Design review of the part built by this model. Coordinates are the model's own, in mm. Face numbers are marked on the shaded views. Round coordinates to 2 decimals unless told otherwise and drop trailing zeros. Loops run counter-clockwise (first coordinate to the right, second up) from the corner with the lowest first, then second, coordinate; pieces in that order, holes last. Notation, with made-up numbers: (-32, 4.25) -> (-20, 4.25) arc R13 cw to (-20, 9.25) -> close; hole circle Ø3 at (46, 52). An arc over 180 degrees is marked (long way). Write each question's results on one line, items separated by ' | '. Start each with the question number.
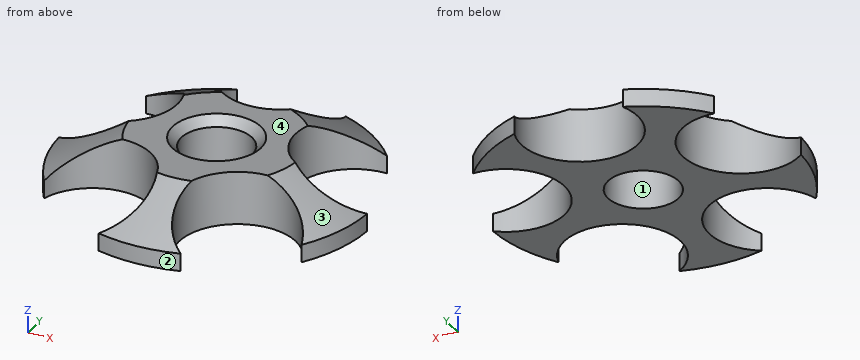
from build123d import *

# Parameters (mm, degrees)
F0_R     = 2
F1_DEPTH = 3
F2_SIZE2 = 2
F2_SIZE  = 4
F3_SIZE  = 0.5


with BuildPart() as f1:
    # F0 (on Top) → F1 (new body)
    with BuildSketch(Plane.XY):
        with BuildLine():
            ThreePointArc((-6.8389636709, 5.4581201808), (-3.5189091103, 1.1433628792), (-8.7410403812, -0.3958699968))
            ThreePointArc((-8.7410403812, -0.3958699968), (-8.3217445176, -2.7038987008), (-7.3043367629, -4.8175890707))
            ThreePointArc((-7.3043367629, -4.8175890707), (-2.1748054335, -2.9933628792), (-2.3246352862, -8.4355539703))
            ThreePointArc((-2.3246352862, -8.4355539703), (0, -8.75), (2.3246352862, -8.4355539703))
            ThreePointArc((2.3246352862, -8.4355539703), (2.1748054335, -2.9933628792), (7.3043367629, -4.8175890707))
            ThreePointArc((7.3043367629, -4.8175890707), (8.3217445176, -2.7038987008), (8.7410403812, -0.3958699968))
            ThreePointArc((8.7410403812, -0.3958699968), (3.5189091103, 1.1433628792), (6.8389636709, 5.4581201808))
            ThreePointArc((6.8389636709, 5.4581201808), (5.1431209576, 7.0788987008), (3.0776247664, 8.1908928571))
            ThreePointArc((3.0776247664, 8.1908928571), (0, 3.7), (-3.0776247664, 8.1908928571))
            ThreePointArc((-3.0776247664, 8.1908928571), (-5.1431209576, 7.0788987008), (-6.8389636709, 5.4581201808))
        make_face()
        Circle(F0_R, mode=Mode.SUBTRACT)
    extrude(amount=F1_DEPTH)

    # F2
    f2_edges = [f1.edges().sort_by_distance(p)[0] for p in [
        (-8.321745, -2.703899, 3),
        (0, -8.75, 3),
        (8.321745, -2.703899, 3),
        (5.143121, 7.078899, 3),
        (-5.143121, 7.078899, 3),
    ]]
    f2_side = f1.faces().sort_by_distance((0, 3.456563, 3))[0]
    chamfer(f2_edges, length=F2_SIZE, length2=F2_SIZE2, reference=f2_side)

    # F3
    f3_edges = [f1.edges().sort_by_distance(p)[0] for p in [
        (-2, 0, 3),
    ]]
    chamfer(f3_edges, length=F3_SIZE)


solid = f1.part
1) Take a section at B-B (y = 0). Write out the cut boundary in (x, z), plus the area to 3 significant figures.
2) To check wall thickness, follow line 1 (Y direction, x = 1.75, z = 0.2); line 2 (Y direction, x = 4, z = 1.4); line 3 (X direction, y = 1.5, z = 2.15). State the ranges of each line that lie inside material, in increasing order. Write a range as from..to.
3) Take a section at A-A (x = 0). Write out the cut boundary in (y, z).
4) The part is to be moulded in two halves that separate along X. For the marked faces 1, 2, 3 and 4, say which applies: +X half, -X half, draft (parallel to the pull), parting line (faces both ways), or undercut.
5) Insertion check: pin 1 (3.5 mm diameter, centred on x = 0, y = 0, fed in from -Z); pin 2 (8.5 mm diameter, centred on x = -4.11, y = -5.66, fed in from -Z); pin 3 (5 mm diameter, centred on x = -6, y = 4.5, fed in from +Z). Each pin has a flat end and moves straight along its axis. Give the tip position at first contact, or say it passes through.
6) Take a section at C-C (z = 2.2). Write out the cut boundary in (x, y), plus the area to 3 significant figures.
Geometry check:
1) outline: (-4.17, 0) -> (-2, 0) -> (-2, 2.5) -> (-2.5, 3) -> (-4.17, 3) -> close; (2, 0) -> (4.17, 0) -> (4.17, 3) -> (2.5, 3) -> (2, 2.5) -> close | area: 12.7 mm^2
2) line 1: y = -8.57..-7.97, -3.36..-0.97, 0.97..4.2 | line 2: y = -2.37..0.21, 4.12..6.87 | line 3: x = -3.42..-1.32, 1.32..3.42
3) outline: (-8.75, 0) -> (-2, 0) -> (-2, 2.5) -> (-2.5, 3) -> (-4.75, 3) -> (-8.75, 1) -> close; (2, 0) -> (3.7, 0) -> (3.7, 3) -> (2.5, 3) -> (2, 2.5) -> close
4) face 1: undercut | face 2: parting line | face 3: +X half | face 4: draft
5) pin 1: passes through | pin 2: stops at z = 0 | pin 3: stops at z = 2.81
6) outline: (-6.25, -1.11) arc R6.35 ccw to (-5.71, -2.78) arc R3.3 cw to (-0.87, -6.29) arc R6.35 ccw to (0.87, -6.29) arc R3.3 cw to (5.71, -2.78) arc R6.35 ccw to (6.25, -1.11) arc R3.3 cw to (4.4, 4.57) arc R6.35 ccw to (2.99, 5.6) arc R3.3 cw to (-2.99, 5.6) arc R6.35 ccw to (-4.4, 4.57) arc R3.3 cw to start; hole circle Ø4 at (0, 0) | area: 58.2 mm^2
